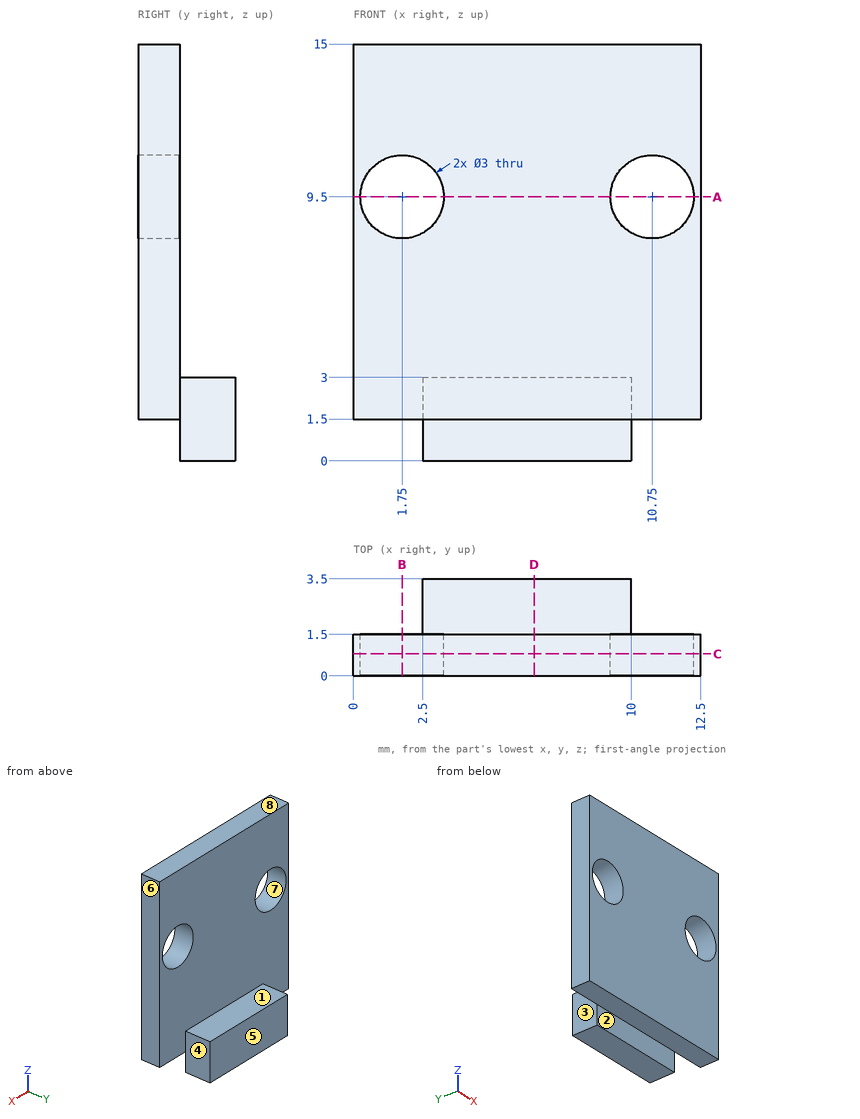
Could you check a few things on this drawing? It's one solid part, dimensions in mm from its lowest x, y, z. A direction names the side the tool comes from. Round coordinates to 2 decimals unless told otherwise and drop trailing zeros. Loops run counter-clockwise (first coordinate to the right, second up) from the corner with the lowest first, then second, coordinate; pieces in that order, holes last. Notation, with made-up numbers: (27.25, 61.5) -> (33.25, 61.5) arc R31 cw to (33.25, 91.5) -> close; hole circle Ø3 at (62, -19). An arc over 180 degrees is marked (long way). Answer as CSV lines item,"result".
1. If we section it at B-B on x = 1.75: Please give me the cut outline in (y, z), plus the area to 4 significant figures.
Final values:
outline,"(0, 1.5) -> (1.5, 1.5) -> (1.5, 8) -> (0, 8) -> close; (0, 11) -> (1.5, 11) -> (1.5, 15) -> (0, 15) -> close"
area,"15.75 mm^2"
2. If I drill on L1, parallel to X at y = 1.1, z = 9.5; L2, parallel to Y at x = 11.75, z = 4.75; L3, parallel to Z at x = 11, y = 0.6, over which ranges is the centre line in solid material (lowest first)?
Final values:
L1,"x = 0 to 0.25, 3.25 to 9.25, 12.25 to 12.5"
L2,"y = 0 to 1.5"
L3,"z = 1.5 to 8.02, 10.98 to 15"
3. Thinking about a two-plate mould opening in X: for the marked faces 6, 7 and 8, which applies, released by +X, released by -X, zero draft, split by the parting line, or undercut?
Final values:
face 6,"released by +X"
face 7,"undercut"
face 8,"zero draft"
4. Which directions (+Z, -Z, +X, -X, +Y, -Y) give clear straight access to the entire face, cutting with the end or side of a thin tool? Please do the marked faces 1, 2, 3, 4 and 5.
Final values:
face 1,"+Z, +X, -X, +Y"
face 2,"-Z, +X, -X, -Y"
face 3,"+Z, -Z, -X, +Y"
face 4,"+Z, -Z, +X, +Y"
face 5,"+Z, -Z, +X, -X, +Y"
5. If we section it at A-A on z = 9.5: Please give me the cut outline in (x, y), plus the area to 3 significant figures.
Final values:
outline,"(0, 0) -> (0.25, 0) -> (0.25, 1.5) -> (0, 1.5) -> close; (3.25, 0) -> (9.25, 0) -> (9.25, 1.5) -> (3.25, 1.5) -> close; (12.25, 0) -> (12.5, 0) -> (12.5, 1.5) -> (12.25, 1.5) -> close"
area,"9.75 mm^2"
6. If we section it at D-D on x = 6.5: Please give me the cut outline in (y, z).
Final values:
outline,"(0, 1.5) -> (1.5, 1.5) -> (1.5, 0) -> (3.5, 0) -> (3.5, 3) -> (1.5, 3) -> (1.5, 15) -> (0, 15) -> close"
7. If we section it at C-C on y = 0.8: Please give me the cut outline in (x, z).
Final values:
outline,"(0, 1.5) -> (12.5, 1.5) -> (12.5, 15) -> (0, 15) -> close; hole circle Ø3 at (1.75, 9.5); hole circle Ø3 at (10.75, 9.5)"
8. For pin 1 (6 mm diameter, centred on x = 4, z = 8.5, fed in from +Y); pin 2 (1 mm diameter, centred on y = 2.5, z = 2, fed in from +X); pin 3 (0.6 mm diameter, centred on y = 2.5, z = 2, fed in from -X), each with a flat end and sliding along its axis, tell me the tip position at first contact or that it passes through.
Final values:
pin 1,"stops at y = 1.5"
pin 2,"stops at x = 10"
pin 3,"stops at x = 2.5"
